Source: CAD feature listing. Evaluate the final solid. Frame: model axes, mm. A direction names the side the tool comes from. Give positions to 0.01 mm unless a question says otherwise; leave off trailing zeros. Order: outer loops, then holes, each group sorted by start corner. A loop starts at its lowest first (then second) coordinate and runs counter-clockwise, first axis right, second up.
```python
from build123d import *

# Parameters (mm, degrees)
RESSALTO_EXTRUS_O1_DEPTH = 1.65
ESBO_O2_W                = 15.5
ESBO_O2_H                = 1.5
RESSALTO_EXTRUS_O2_DEPTH = 3
ESBO_O3_W                = 1.5
ESBO_O3_H                = 9.5
RESSALTO_EXTRUS_O3_DEPTH = 2
ESBO_O4_R                = 5.25
CORTE_EXTRUS_O1_DEPTH    = 26.913997794
FILETE1_R                = 2
CHANFRO1_SIZE            = 0.352653961
CHANFRO1_SIZE_2          = 2
FILETE3_R                = 2
FILETE4_R                = 1
FILETE5_R                = 1
FILETE6_R                = 1
FILETE7_R                = 1


with BuildPart() as part:
    # Esboço1 → Ressalto-extrusão1 (new body)
    with BuildSketch(Plane(origin=(0, 0, 0), x_dir=(1, 0, 0), z_dir=(0, 1, 0))):
        Polygon((-9.875, 2.10086556), (9.875, 2.10086556), (10.75, -8.49913444), (14, -8.49913444), (14, -17.99913444), (7.75, -17.99913444), (7.75, -21.49913444), (-7.75, -21.49913444), (-7.75, -17.99913444), (-14, -17.99913444), (-14, -8.49913444), (-10.75, -8.49913444), align=None)
    extrude(amount=RESSALTO_EXTRUS_O1_DEPTH)

    # Esboço2 → Ressalto-extrusão2 (add)
    with BuildSketch(Plane(origin=(0, 1.65, 0), x_dir=(1, 0, 0), z_dir=(0, 1, 0))):
        with Locations((0, -20.74913444)):
            Rectangle(ESBO_O2_W, ESBO_O2_H)
    extrude(amount=RESSALTO_EXTRUS_O2_DEPTH)

    # Esboço3 → Ressalto-extrusão3 (add)
    with BuildSketch(Plane.XZ):
        with Locations((-13.25, 13.24913444)):
            Rectangle(ESBO_O3_W, ESBO_O3_H)
        with Locations((13.25, 13.24913444)):
            Rectangle(ESBO_O3_W, ESBO_O3_H)
    extrude(amount=RESSALTO_EXTRUS_O3_DEPTH)

    # Esboço4 → Corte-extrusão1 (cut, through all)
    with BuildSketch(Plane(origin=(0, 1.65, 0), x_dir=(1, 0, 0), z_dir=(0, 1, 0))):
        with Locations(Location((0, -9.89913444, 0), (0, 0, 270))):
            Circle(ESBO_O4_R)
    extrude(amount=-CORTE_EXTRUS_O1_DEPTH, mode=Mode.SUBTRACT)

    # Filete1
    filete1_edges = [part.edges().sort_by_distance(p)[0] for p in [
        (14, 1.65, 13.24913444),
        (-14, 1.65, 13.24913444),
    ]]
    fillet(filete1_edges, radius=FILETE1_R)

    # Chanfro1
    # the kernel refuses this chamfer: 2, 0.352653961 mm, written as the material it adds along each edge
    with BuildSketch(Plane(origin=(12.5, 0, 17.99913444), x_dir=(-0.9776715712462587, 0.21013876076743104, 0), z_dir=(0, 0, -1))) as chanfro1_piece_1_section:
        Polygon((CHANFRO1_SIZE * 0.977671572402, -CHANFRO1_SIZE * 0.210138761016), (-CHANFRO1_SIZE_2 * 0.210138760767, -CHANFRO1_SIZE_2 * 0.977671571246), (0, 0), align=None)
    chanfro1_piece_1 = extrude(amount=9.5, mode=Mode.PRIVATE)
    chanfro1_piece_1 = split(chanfro1_piece_1, bisect_by=Plane(origin=(12.403792596, -2, 13.24913444), z_dir=(0, 1, 0)), keep=Keep.TOP, mode=Mode.PRIVATE)
    add(chanfro1_piece_1)
    with BuildSketch(Plane(origin=(-12.5, 0, 17.99913444), x_dir=(0.9776715712462587, 0.21013876076743104, 0), z_dir=(0, 0, -1))) as chanfro1_piece_2_section:
        Polygon((CHANFRO1_SIZE * 0.977671572402, CHANFRO1_SIZE * 0.210138761016), (-CHANFRO1_SIZE_2 * 0.210138760767, CHANFRO1_SIZE_2 * 0.977671571246), (0, 0), align=None)
    chanfro1_piece_2 = extrude(amount=9.5, mode=Mode.PRIVATE)
    chanfro1_piece_2 = split(chanfro1_piece_2, bisect_by=Plane(origin=(-12.403792596, -2, 13.24913444), z_dir=(0, 1, 0)), keep=Keep.TOP, mode=Mode.PRIVATE)
    add(chanfro1_piece_2)

    # Filete3
    filete3_edges = [part.edges().sort_by_distance(p)[0] for p in [
        (0, 0, 21.49913444),
    ]]
    fillet(filete3_edges, radius=FILETE3_R)

    # Filete4
    filete4_edges = [part.edges().sort_by_distance(p)[0] for p in [
        (0, 1.65, 19.99913444),
    ]]
    fillet(filete4_edges, radius=FILETE4_R)

    # Filete5
    filete5_edges = [part.edges().sort_by_distance(p)[0] for p in [
        (-9.875, 0.825, -2.10086556),
    ]]
    fillet(filete5_edges, radius=FILETE5_R)

    # Filete6
    filete6_edges = [part.edges().sort_by_distance(p)[0] for p in [
        (9.875, 0.825, -2.10086556),
    ]]
    fillet(filete6_edges, radius=FILETE6_R)

    # Filete7
    filete7_edges = [part.edges().sort_by_distance(p)[0] for p in [
        (-10.75, 0.825, 8.49913444),
        (-7.75, 0.825, 17.99913444),
        (7.75, 0.825, 17.99913444),
        (10.75, 0.825, 8.49913444),
    ]]
    fillet(filete7_edges, radius=FILETE7_R)


solid = part.part
```
1) Pin query (flat end, axial travel): pin 1 (0.7 mm diameter, centred on x = 12.5, y = 0.5, fed in from -Z); pin 2 (6.5 mm diameter, centred on x = 5.5, z = 7, fed in from +Y); pin 3 (13.5 mm diameter, centred on x = 0, z = 9.9, fed in from -Y). Return the tip coordinate at first contact, or that it passes through.
Report:
pin 1: stops at z = 8.5
pin 2: stops at y = 1.65
pin 3: stops at y = 0
2) Draft query along X for faces 1 (the flat face through (12.32, -0.99, 13.32)), 2 (the cylindrical face through (0.231, 0.837, 4.654)), 3 (the flat face through (-14, -1, 13)), 4 (the cylindrical face through (9.624, 0.837, -1.844)). Return one class per face: +X half, -X half, draft (parallel to the pull), parting line (faces both ways), or undercut.
Report:
face 1: undercut
face 2: undercut
face 3: -X half
face 4: +X half
3) Section query C-C, the plane y = 4.25. Return the cut outline in (x, z), and give its area (4 significant figures).
Report:
outline: (-7.75, 20) - (7.75, 20) - (7.75, 21.5) - (-7.75, 21.5) - close
area: 23.25 mm2
4) Section query A-A, the plane x = 0. Return the cut outline in (y, z), and give its area (3 significant figures).
Report:
outline: (0, -2.1) - (1.65, -2.1) - (1.65, 4.65) - (0, 4.65) - close; (0, 15.15) - (1.65, 15.15) - (1.65, 19) arc R1 cw to (2.65, 20) - (4.65, 20) - (4.65, 21.5) - (2, 21.5) arc R2 ccw to (0, 19.5) - close
area: 25.5 mm2
5) Reachability of faces 5 (the flat face through (7.75, 2, 21)), 6 (the flat face through (-13, 0, 8.499)), 7 (the flat face through (-11.5, 0.4, 17.999)) from +Z, -Z, +X, -X, +Y, -Y: full face, straight path, thin tool, end or side. Return the list, or none.
Report:
face 5: +Z, +X, +Y, -Y
face 6: -Z, -X, +Y, -Y
face 7: +Z, -X, +Y, -Y
6) Material intervals for L1, parallel to Y at x = 5.25, z = 19; L2, parallel to X at y = -1, z = 15.5, sorted ascending.
Report:
L1: y = 0 to 1.65
L2: x = -14 to -12.32, 12.32 to 14
7) Section query B-B, the plane z = 6.75. Return the cut outline in (x, y), and give its area (3 significant figures).
Report:
outline: (-10.61, 0) - (-4.2, 0) - (-4.2, 1.65) - (-10.61, 1.65) - close; (4.2, 0) - (10.61, 0) - (10.61, 1.65) - (4.2, 1.65) - close
area: 21.1 mm2
8) Section query D-D, the plane z = 16.75. Return the cut outline in (x, y).
Report:
outline: (-14, -2) - (-12.5, -2) - (-12.15, 0) - (12.15, 0) - (12.5, -2) - (14, -2) - (14, -0.35) arc R2 ccw to (12, 1.65) - (-12, 1.65) arc R2 ccw to (-14, -0.35) - close
